For this review, take the finished solid that the model builds, in its own axes (mm). Face numbers are marked on the shaded views. A direction names the side the tool comes from. Give positions to 0.01 mm unless a question says otherwise; leave off trailing zeros. Loops run counter-clockwise (first coordinate to the right, second up) from the corner with the lowest first, then second, coordinate; pieces in that order, holes last. Notation, with made-up numbers: (69.25, -30.75) - (86.25, -30.75) arc R30 ccw to (86.25, -2.75) - close; hole circle Ø7 at (-9, 54.25). An arc over 180 degrees is marked (long way). Answer in a Markdown table with one row per item.
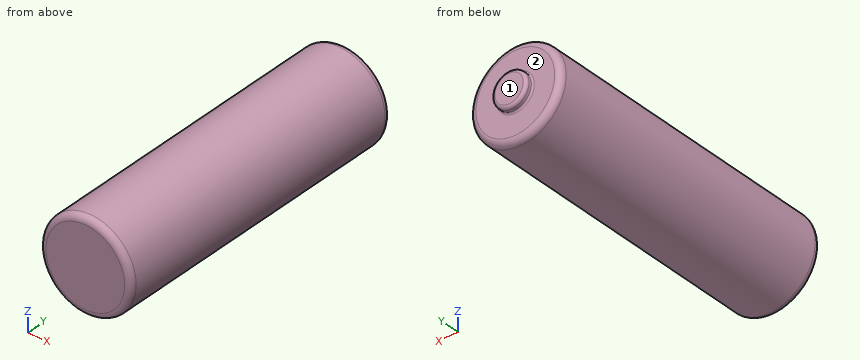
```python
from build123d import *

# Parameters (mm, degrees)
SKETCH1_R           = 7.25
BOSS_EXTRUDE4_DEPTH = 49.5
SKETCH8_R           = 2.75
BOSS_EXTRUDE5_DEPTH = 1.2
FILLET1_R           = 1
FILLET3_R           = 0.25
FILLET4_R           = 0.5


with BuildPart() as part:
    # Sketch1 → Boss-Extrude4 (new body)
    with BuildSketch(Plane(origin=(0, 0, 0), x_dir=(1, 0, 0), z_dir=(0, 1, 0))):
        with Locations(Location((0, 0, 0), (0, 0, 270))):
            Circle(SKETCH1_R)
    extrude(amount=BOSS_EXTRUDE4_DEPTH)

    # Sketch8 → Boss-Extrude5 (add)
    with BuildSketch(Plane(origin=(0, 49.5, 0), x_dir=(1, 0, 0), z_dir=(0, 1, 0))):
        with Locations(Location((0, 0, 0), (0, 0, 270))):
            Circle(SKETCH8_R)
    extrude(amount=BOSS_EXTRUDE5_DEPTH)

    # Fillet1
    fillet1_edges = [part.edges().sort_by_distance(p)[0] for p in [
        (0, 0, -7.25),
        (0, 49.5, -7.25),
    ]]
    fillet(fillet1_edges, radius=FILLET1_R)

    # Fillet3
    fillet3_edges = [part.edges().sort_by_distance(p)[0] for p in [
        (0, 49.5, -2.75),
    ]]
    fillet(fillet3_edges, radius=FILLET3_R)

    # Fillet4
    fillet4_edges = [part.edges().sort_by_distance(p)[0] for p in [
        (0, 50.7, -2.75),
    ]]
    fillet(fillet4_edges, radius=FILLET4_R)


solid = part.part
```
1. Wall thickness on line 1 (Y direction, x = 3.5, z = 4); line 2 (Y direction, x = -1.75, z = -1.5); line 3 (Z direction, x = -5.75, y = 41.5): over which ranges is each line inside the solid? List them lowest first. Write a range as [from, to].
Values:
| item | result |
|---|---|
| line 1 | y = [0, 49.5] |
| line 2 | y = [0, 50.7] |
| line 3 | z = [-4.42, 4.42] |
2. We need section A-A, the plane x = 0. Give the boundary of the cut face in (y, z).
Values:
| item | result |
|---|---|
| outline | (0, -6.25) arc R1 ccw to (1, -7.25) - (48.5, -7.25) arc R1 ccw to (49.5, -6.25) - (49.5, -3) arc R0.25 cw to (49.75, -2.75) - (50.2, -2.75) arc R0.5 ccw to (50.7, -2.25) - (50.7, 2.25) arc R0.5 ccw to (50.2, 2.75) - (49.75, 2.75) arc R0.25 cw to (49.5, 3) - (49.5, 6.25) arc R1 ccw to (48.5, 7.25) - (1, 7.25) arc R1 ccw to (0, 6.25) - close |
3. We need section C-C, the plane y = 38. Give the boundary of the cut face in (x, z).
Values:
| item | result |
|---|---|
| outline | circle Ø14.5 at (0, 0) |
4. Clearance check with flat-ended pins moving along their axes: pin 1 (1 mm diameter, centred on y = 20.5, z = -2.5, fed in from +X); pin 2 (1 mm diameter, centred on y = 26.5, z = -4.5, fed in from +X); pin 3 (1.5 mm diameter, centred on x = -4.5, y = 27, fed in from +Z). State where each tip first meets the part, or that it passes through.
Values:
| item | result |
|---|---|
| pin 1 | stops at x = 6.97 |
| pin 2 | stops at x = 6.05 |
| pin 3 | stops at z = 6.2 |
5. For the marked faces 1 and 2, list the 3-axis set-ups (+Z, -Z, +X, -X, +Y, -Y) from which the entire face can be reached by the end or side of a thin tool; tool diameter is ignored.
Values:
| item | result |
|---|---|
| face 1 | +Z, -Z, +X, -X, +Y |
| face 2 | +Y |
6. We need section B-B, the plane z = 0. Give the boundary of the cut face in (x, y), and give its area (3 significant figures).
Values:
| item | result |
|---|---|
| outline | (-7.25, 1) arc R1 ccw to (-6.25, 0) - (6.25, 0) arc R1 ccw to (7.25, 1) - (7.25, 48.5) arc R1 ccw to (6.25, 49.5) - (3, 49.5) arc R0.25 cw to (2.75, 49.75) - (2.75, 50.2) arc R0.5 ccw to (2.25, 50.7) - (-2.25, 50.7) arc R0.5 ccw to (-2.75, 50.2) - (-2.75, 49.75) arc R0.25 cw to (-3, 49.5) - (-6.25, 49.5) arc R1 ccw to (-7.25, 48.5) - close |
| area | 723 mm^2 |
